```python
from build123d import *

# Parameters (mm, degrees)
SALIENTE_EXTRUIR1_DEPTH = 4
REDONDEO1_R             = 5
CROQUIS2_W              = 3
CROQUIS2_H              = 6
SALIENTE_EXTRUIR2_DEPTH = 22.44
REDONDEO2_R             = 25
CROQUIS3_R              = 0.5
CORTAR_EXTRUIR1_DEPTH   = 2
REDONDEO3_R             = 1


with BuildPart() as part:
    # Croquis1 → Saliente-Extruir1 (new body)
    # profile 1 of 4: a face of its own
    with BuildSketch(Plane.XY):
        with BuildLine():
            Line((-38, -3.5), (-38, -8.5))
            ThreePointArc((-38, -8.5), (-41.5, -12), (-45, -8.5))
            Line((-45, -8.5), (-45, -3.5))
            ThreePointArc((-45, -3.5), (-41.5, 0), (-38, -3.5))
        make_face()
        with BuildLine():
            ThreePointArc((-44, -8.5), (-41.5, -11), (-39, -8.5))
            Line((-39, -8.5), (-39, -3.5))
            ThreePointArc((-39, -3.5), (-41.5, -1), (-44, -3.5))
            Line((-44, -3.5), (-44, -8.5))
        make_face(mode=Mode.SUBTRACT)
    # profile 2 of 4: a face of its own
    with BuildSketch(Plane.XY):
        with BuildLine():
            Line((0, 0), (-41.5, 0))
            ThreePointArc((-41.5, 0), (-39.025126266, -1.025126266), (-38, -3.5))
            Line((-38, -3.5), (-38, -6))
            Line((-38, -6), (0, -6))
            Line((0, -6), (0, 0))
        make_face()
    # profile 3 of 4: a face of its own
    with BuildSketch(Plane.XY):
        with BuildLine():
            Line((41.5, 0), (0, 0))
            Line((0, 0), (0, -6))
            Line((0, -6), (38, -6))
            Line((38, -6), (38, -3.5))
            ThreePointArc((38, -3.5), (39.025126266, -1.025126266), (41.5, 0))
        make_face()
    # profile 4 of 4: a face of its own
    with BuildSketch(Plane.XY):
        with BuildLine():
            ThreePointArc((45, -8.5), (41.5, -12), (38, -8.5))
            Line((38, -8.5), (38, -3.5))
            ThreePointArc((38, -3.5), (41.5, 0), (45, -3.5))
            Line((45, -3.5), (45, -8.5))
        make_face()
        with BuildLine():
            Line((39, -3.5), (39, -8.5))
            ThreePointArc((39, -8.5), (41.5, -11), (44, -8.5))
            Line((44, -8.5), (44, -3.5))
            ThreePointArc((44, -3.5), (41.5, -1), (39, -3.5))
        make_face(mode=Mode.SUBTRACT)
    extrude(amount=SALIENTE_EXTRUIR1_DEPTH)

    # Redondeo1
    redondeo1_edges = [part.edges().sort_by_distance(p)[0] for p in [
        (38, -6, 2),
        (-38, -6, 2),
    ]]
    fillet(redondeo1_edges, radius=REDONDEO1_R)

    # Croquis2 → Saliente-Extruir2 (add)
    with BuildSketch(Plane.XY.offset(4)):
        with Locations((0, -3)):
            Rectangle(CROQUIS2_W, CROQUIS2_H)
    extrude(amount=SALIENTE_EXTRUIR2_DEPTH)

    # Redondeo2
    # the kernel refuses this fillet: 25 mm, written as the material it adds along each edge
    with BuildSketch(Plane(origin=(1.5, -6, 4), x_dir=(1, 0, 0), z_dir=(0, 1, 0)), Plane(origin=(-1.5, 0, 4), x_dir=(-1, 0, 0), z_dir=(0, -1, 0))) as redondeo2_piece_1:
        with BuildLine():
            CenterArc((24.868582589, -25), REDONDEO2_R, 90, 84.122610013)
            Line((0, -22.44), (-0.497371652, -22.3888))
            ThreePointArc((-0.497371652, -22.3888), (-0.5, -11.22), (-0.5, 0))
            Line((-0.5, 0), (0, 0.5))
            Line((0, 0.5), (24.868582589, 0.5))
            Line((24.868582589, 0.5), (24.868582589, 0))
        make_face()
    extrude(amount=6)

    # Croquis3 → Cortar-Extruir1 (cut)
    with BuildSketch(Plane.XY.offset(26.44)):
        with Locations((0, -3)):
            Circle(CROQUIS3_R)
    extrude(amount=-CORTAR_EXTRUIR1_DEPTH, mode=Mode.SUBTRACT)

    # Redondeo3
    redondeo3_edges = [part.edges().sort_by_distance(p)[0] for p in [
        (-1.5, -3, 26.44),
        (1.5, -3, 26.44),
    ]]
    fillet(redondeo3_edges, radius=REDONDEO3_R)


solid = part.part
```
Verification items for the finished model (mm, model axes). A direction names the side the tool comes from. Give positions to 0.01 mm unless a question says otherwise; leave off trailing zeros. Loops run counter-clockwise (first coordinate to the right, second up) from the corner with the lowest first, then second, coordinate; pieces in that order, holes last.
1. Thickness scan on line 1 (Y direction, x = 0, z = 25.5); line 2 (Y direction, x = 0.5, z = 17); line 3 (Z direction, x = -38, y = -3). Record the ranges inside material, lowest first.
2. Section check B-B, the plane x = -29.5. Enter the section's corners in (y, z).
3. Section check C-C, the plane z = 14.5. Enter the section's corners in (x, y), then the cut area to 3 significant figures.
4. Go/stop test with flat-tipped pins: pin 1 Ø2 at (x, y) = (6.5, -8.5) entering from -Z; pin 2 Ø3.5 at (x, y) = (38, -7.5) entering from +Z; pin 3 Ø10 at (x, z) = (7.5, 3.5) entering from -Y. Record where each tip stops, or that it passes through.
5. Set-up check for faces 1 (the flat face through (0, -6, 7)), 2 (the flat face through (-39, -6, 2)), 3 (the flat face through (36, -5, 4)): record each of +Z, -Z, +X, -X, +Y, -Y from which the full face is reachable in a straight line by a thin tool's end or side.
6. Section check A-A, the plane y = -4.5. Enter the section's corners in (x, z), then the cut area to 3 significant figures.
7. Mould release check, pull along X, two halves, no side actions. Record for faces 4 (the flat face through (-33, -3, 4)), 5 (the flat face through (-44, -6, 2)), 6 (the cylindrical face through (-10.136, -2.958, 9.987)): released by +X, released by -X, zero draft, split by the parting line, or undercut.
Geometry says:
1. line 1: y = -6 to -3.5, -2.5 to 0
1. line 2: y = -6 to 0
1. line 3: z = 0 to 4
2. outline: (-6, 0) - (0, 0) - (0, 4) - (-6, 4) - close
3. outline: (-6, -6) - (6, -6) - (6, 0) - (-6, 0) - close
3. area: 72.0 mm2
4. pin 1: passes through
4. pin 2: stops at z = 4
4. pin 3: stops at y = -6
5. face 1: +Z, -Z, -Y
5. face 2: +Z, -Z
5. face 3: +Z, +X, +Y, -Y
6. outline: (-45, 0) - (-44, 0) - (-44, 4) - (-45, 4) - close; (-39, 0) - (39, 0) - (39, 4) - (26.37, 4) arc R25 cw to (1.6, 25.58) arc R1 ccw to (0.61, 26.44) - (-0.61, 26.44) arc R1 ccw to (-1.6, 25.58) arc R25 cw to (-26.37, 4) - (-39, 4) - close; (44, 0) - (45, 0) - (45, 4) - (44, 4) - close
6. area: 649 mm2
7. face 4: zero draft
7. face 5: undercut
7. face 6: released by -X
